The listing builds one solid part. Answer for the finished solid, in the listing's coordinates (mm). Face numbers are marked on the shaded views. A direction names the side the tool comes from. Coordinates: 2 decimals unless noted, no trailing zeros. Order: outer loops, then holes, each group sorted by start corner. A loop starts at its lowest first (then second) coordinate and runs counter-clockwise, first axis right, second up. Notation, with made-up numbers: (61.5, -18.5) -> (83.5, -18.5) arc R26 cw to (83.5, -1.5) -> close; hole circle Ø4 at (76.5, 11). An arc over 180 degrees is marked (long way). Return JSON: item names as keys, results as strings.
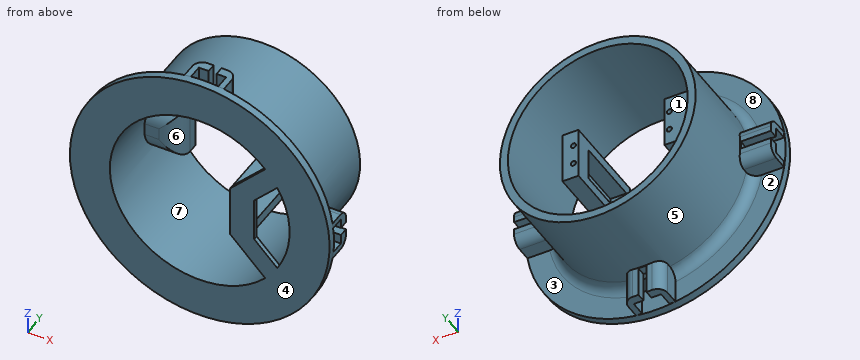
```python
from build123d import *

# Parameters (mm, degrees)
CROQUIS1_R              = 49
CROQUIS1_R_2            = 45
SALIENTE_EXTRUIR1_DEPTH = 56
CROQUIS3_R              = 65
CROQUIS3_R_2            = 49
SALIENTE_EXTRUIR2_DEPTH = 4
REDONDEO1_R             = 5
CROQUIS4_W              = 8
CROQUIS4_H              = 26
SALIENTE_EXTRUIR3_DEPTH = 46
SALIENTE_EXTRUIR4_DEPTH = 2.2
SALIENTE_EXTRUIR5_START = -15
SALIENTE_EXTRUIR5_DEPTH = 15
REDONDEO2_R             = 10
CROQUIS7_R              = 1.3
CORTAR_EXTRUIR1_DEPTH   = 7.2
CORTAR_EXTRUIR2_REACH   = 119.478
CROQUIS8_W              = 16
CROQUIS8_H              = 34
CROQUIS9_W              = 16.249513617
CROQUIS9_H              = 19.697715604
SALIENTE_EXTRUIR6_DEPTH = 12
REDONDEO3_R             = 5
CROQUIS11_W             = 13.697715604
CROQUIS11_H             = 7.5
CORTAR_EXTRUIR3_DEPTH   = 12
CROQUIS12_W             = 4
CROQUIS12_H             = 4.5
CORTAR_EXTRUIR4_DEPTH   = 15
MATRIZC1_COUNT          = 4
REDONDEO3_OF_MATRIZC1_R = 5


with BuildPart() as part:
    # Croquis1 → Saliente-Extruir1 (new body)
    with BuildSketch(Plane(origin=(0, 0, 0), x_dir=(1, 0, 0), z_dir=(0, 1, 0))):
        with Locations(Location((0, 0, 0), (0, 0, 270))):
            Circle(CROQUIS1_R)
        with Locations(Location((0, 0, 0), (0, 0, 270))):
            Circle(CROQUIS1_R_2, mode=Mode.SUBTRACT)
    extrude(amount=SALIENTE_EXTRUIR1_DEPTH)

    # Croquis3 → Saliente-Extruir2 (add)
    with BuildSketch(Plane(origin=(0, 0, 0), x_dir=(1, 0, 0), z_dir=(0, 1, 0))):
        with Locations(Location((0, 0, 0), (0, 0, 270))):
            Circle(CROQUIS3_R)
        with Locations(Location((0, 0, 0), (0, 0, 270))):
            Circle(CROQUIS3_R_2, mode=Mode.SUBTRACT)
    extrude(amount=SALIENTE_EXTRUIR2_DEPTH)

    # Redondeo1
    redondeo1_edges = [part.edges().sort_by_distance(p)[0] for p in [
        (0, 4, -49),
    ]]
    fillet(redondeo1_edges, radius=REDONDEO1_R)



with BuildPart() as body_2:
    # Croquis4 → Saliente-Extruir3 (new body)
    with BuildSketch(Plane(origin=(0, 0, 0), x_dir=(1, 0, 0), z_dir=(0, 1, 0))):
        with Locations((19.25, 0)):
            Rectangle(CROQUIS4_W, CROQUIS4_H)
    extrude(amount=SALIENTE_EXTRUIR3_DEPTH)


with BuildPart() as part_1:
    add(part.part)

    add(body_2.part)  # Saliente-Extruir4 merges body 2
    # Croquis5 → Saliente-Extruir4 (add)
    with BuildSketch(Plane(origin=(0, 0, 0), x_dir=(1, 0, 0), z_dir=(0, 1, 0))):
        with BuildLine():
            Line((15.25, 13), (32.749541701, 30.86207249))
            ThreePointArc((32.749541701, 30.86207249), (36.011367089, 26.98483723), (38.816649113, 22.765494759))
            Line((38.816649113, 22.765494759), (27.25, 10.959224145))
            Line((27.25, 10.959224145), (27.25, -10.959224145))
            Line((27.25, -10.959224145), (38.816649113, -22.765494759))
            ThreePointArc((38.816649113, -22.765494759), (36.011367089, -26.98483723), (32.749541701, -30.86207249))
            Line((32.749541701, -30.86207249), (15.25, -13))
            Line((15.25, -13), (23.25, -13))
            Line((23.25, -13), (23.25, 13))
            Line((23.25, 13), (15.25, 13))
        make_face()
    extrude(amount=SALIENTE_EXTRUIR4_DEPTH)

    # Croquis6 → Saliente-Extruir5 (add)
    with BuildSketch(Plane(origin=(0, 46, 0), x_dir=(1, 0, 0), z_dir=(0, 1, 0)).offset(SALIENTE_EXTRUIR5_START)):
        with BuildLine():
            Line((-27.75, 13), (-43.081318457, 13))
            ThreePointArc((-43.081318457, 13), (-45, 0), (-43.081318457, -13))
            Line((-43.081318457, -13), (-27.75, -13))
            Line((-27.75, -13), (-27.75, 13))
        make_face()
    extrude(amount=SALIENTE_EXTRUIR5_DEPTH)

    # Redondeo2
    redondeo2_edges = [part_1.edges().sort_by_distance(p)[0] for p in [
        (-27.75, 31, 0),
        (-35.415659229, 31, 13),
        (-35.415659229, 31, -13),
    ]]
    fillet(redondeo2_edges, radius=REDONDEO2_R)

    # Croquis7 → Cortar-Extruir1 (cut)
    with BuildSketch(Plane(origin=(0, 46, 0), x_dir=(1, 0, 0), z_dir=(0, 1, 0))):
        with Locations(Location((17.75, 5, 0), (0, 0, 270))):
            Circle(CROQUIS7_R)
        with Locations(Location((17.75, -5, 0), (0, 0, 90))):
            Circle(CROQUIS7_R)
        with Locations(Location((-30.25, -5, 0), (0, 0, 270))):
            Circle(CROQUIS7_R)
        with Locations(Location((-30.25, 5, 0), (0, 0, 90))):
            Circle(CROQUIS7_R)
    extrude(amount=-CORTAR_EXTRUIR1_DEPTH, mode=Mode.SUBTRACT)

    # Croquis8 → Cortar-Extruir2 (cut, up to next)
    with BuildSketch(Plane.ZY.offset(-15.25), mode=Mode.PRIVATE) as cortar_extruir2_sk1:
        with Locations((0, 20)):
            Rectangle(CROQUIS8_W, CROQUIS8_H)
    cortar_extruir2_tool1 = extrude(cortar_extruir2_sk1.sketch, amount=-CORTAR_EXTRUIR2_REACH, mode=Mode.PRIVATE) & part_1.part
    add(cortar_extruir2_tool1.solids().sort_by_distance((15.25, 20, 0))[0], mode=Mode.SUBTRACT)

    # Croquis9 → Saliente-Extruir6 (add)
    with BuildSketch(Plane(origin=(0, 4, 0), x_dir=(1, 0, 0), z_dir=(0, 1, 0))):
        with Locations((-56.124756809, 0)):
            Rectangle(CROQUIS9_W, CROQUIS9_H)
    saliente_extruir6 = extrude(amount=SALIENTE_EXTRUIR6_DEPTH)

    # Redondeo3
    redondeo3_edges = [part_1.edges().sort_by_distance(p)[0] for p in [
        (-56.124756808, 16, -9.848857802),
        (-56.124756808, 16, 9.848857802),
    ]]
    fillet(redondeo3_edges, radius=REDONDEO3_R)

    # Croquis11 → Cortar-Extruir3 (cut)
    with BuildSketch(Plane.ZY.offset(64.249513617)):
        with Locations((0, 7.75)):
            Rectangle(CROQUIS11_W, CROQUIS11_H)
    cortar_extruir3 = extrude(amount=-CORTAR_EXTRUIR3_DEPTH, mode=Mode.SUBTRACT)

    # Croquis12 → Cortar-Extruir4 (cut)
    with BuildSketch(Plane.ZY.offset(64.249513617)):
        with Locations((0, 13.75)):
            Rectangle(CROQUIS12_W, CROQUIS12_H)
    cortar_extruir4 = extrude(amount=-CORTAR_EXTRUIR4_DEPTH, mode=Mode.SUBTRACT)

    # MatrizC1: Saliente-Extruir6, Cortar-Extruir3, Cortar-Extruir4 ×4 about axis
    matrizc1_axis = Axis((0, 0, 0), (0, 1, 0))
    add([saliente_extruir6.rotate(matrizc1_axis, i * 360 / MATRIZC1_COUNT) for i in range(1, MATRIZC1_COUNT)])
    add([cortar_extruir3.rotate(matrizc1_axis, i * 360 / MATRIZC1_COUNT) for i in range(1, MATRIZC1_COUNT)], mode=Mode.SUBTRACT)
    add([cortar_extruir4.rotate(matrizc1_axis, i * 360 / MATRIZC1_COUNT) for i in range(1, MATRIZC1_COUNT)], mode=Mode.SUBTRACT)

    # Redondeo3 of MatrizC1
    redondeo3_of_matrizc1_edges = [part_1.edges().sort_by_distance(p)[0] for p in [
        (-9.848857802, 16, 56.124756808),
        (9.848857802, 16, 56.124756808),
        (56.124756808, 16, 9.848857802),
        (56.124756808, 16, -9.848857802),
        (9.848857802, 16, -56.124756808),
        (-9.848857802, 16, -56.124756808),
    ]]
    fillet(redondeo3_of_matrizc1_edges, radius=REDONDEO3_OF_MATRIZC1_R)


solid = part_1.part
```
Item 1: Which of the six approach directions +Z, -Z, +X, -X, +Y, -Y give full straight-line access (tool end or side, diameter ignored) to the marked faces 1, 2, 3 and 4?
Answer list:
{"face 1": "+Y", "face 2": "-Z, -X, +Y", "face 3": "-Z, +X, +Y", "face 4": "+Z, -Z, +X, -X, -Y"}
Item 2: Flat-ended cylindrical pins translate along their axes: pin 1 (3.5 mm diameter, centred on x = 60, y = 13.5, fed in from +Z); pin 2 (1 mm diameter, centred on y = 29, z = 51, fed in from +X); pin 3 (8 mm diameter, centred on y = 12.5, z = 38, fed in from -X); pin 4 (5.5 mm diameter, centred on y = 7, z = 59, fed in from +X). Find the tip coordinate at first contact, or state that the pin passes through.
Answer list:
{"pin 1": "z = 9.79", "pin 2": "through", "pin 3": "x = -35.28", "pin 4": "x = 9.85"}
Item 3: The part is cut by section C-C on x = 0. Determine the outline of the cut face in (y, z).
Answer list:
{"outline": "(0, -65) -> (4, -65) -> (4, -52.25) -> (11.5, -52.25) -> (11.5, -49.25) -> (16, -49.25) -> (16, -49) -> (56, -49) -> (56, -45) -> (0, -45) -> close; (0, 45) -> (56, 45) -> (56, 49) -> (16, 49) -> (16, 49.25) -> (11.5, 49.25) -> (11.5, 52.25) -> (4, 52.25) -> (4, 65) -> (0, 65) -> close"}
Item 4: Determine the mould class of the marked faces 5, 6, 7 and 8 for opening direction Z: pulls with the +Z half, pulls with the -Z half, needs draft (parallel to the pull), parting line crosses it, or undercut.
Answer list:
{"face 5": "parting line crosses it", "face 6": "undercut", "face 7": "undercut", "face 8": "needs draft"}
Item 5: The part is cut by section D-D on z = 0. Count the separate pieces of the cut face and the enclosed holes in it, plus the area to 3 significant figures.
Answer list:
{"separate pieces": "4", "enclosed holes": "0", "area": "969 mm2"}
Item 6: The part is cut by section A-A on y = 43. Determine the outline of the cut face in (x, z), plus the area to 3 significant figures.
Answer list:
{"outline": "circle Ø98 at (0, 0); (15.25, -13) -> (23.25, -13) -> (23.25, 13) -> (15.25, 13) -> close; hole (-43.08, -13) arc R45 ccw (long way) to (-43.08, 13) -> (-27.75, 13) -> (-27.75, -13) -> close; hole circle Ø2.6 at (-30.25, -5); hole circle Ø2.6 at (-30.25, 5); hole circle Ø2.6 at (17.75, -5); hole circle Ø2.6 at (17.75, 5)", "area": "1,800 mm2"}
Item 7: The part is cut by section B-B on y = 23. Determine the outline of the cut face in (x, z).
Answer list:
{"outline": "circle Ø98 at (0, 0); (15.25, -13) -> (23.25, -13) -> (23.25, -8) -> (15.25, -8) -> close; (15.25, 8) -> (23.25, 8) -> (23.25, 13) -> (15.25, 13) -> close; hole circle Ø90 at (0, 0)"}
Item 8: Find the intervals of material crossed by probe 1 along X at (y, z) = (12, 0); probe 2 along Z at (x, y) = (-30, 40); probe 3 along Y at (x, z) = (57, 4), in increasing order.
Answer list:
{"probe 1": "-49.25 to -45, 45 to 49.25", "probe 2": "-38.74 to -33.54, -12.95 to -6.28, -3.72 to 3.72, 6.28 to 12.95, 33.54 to 38.74", "probe 3": "0 to 4, 11.5 to 16"}
